CAD build for the part. Positions are in the model's coordinates, mm. A direction names the side the tool comes from. Coordinates: 2 decimals unless noted, no trailing zeros. Order: outer loops, then holes, each group sorted by start corner. A loop starts at its lowest first (then second) coordinate and runs counter-clockwise, first axis right, second up. Notation, with made-up numbers: (43, 74.25) - (86, 74.25) arc R21 cw to (86, 101.25) - close; hole circle Ø2 at (66, 27). An arc over 180 degrees is marked (long way). Use one line per item in the form item = value.
```python
from build123d import *

# Parameters (mm, degrees)
BOSS_EXTRUDE1_DEPTH = 10
SKETCH2_R           = 1.5
CUT_EXTRUDE1_DEPTH  = 107.852975625
BOSS_EXTRUDE2_DEPTH = 0.5
SKETCH5_R           = 3.25
CUT_EXTRUDE2_DEPTH  = 5
FILLET1_R           = 15


with BuildPart() as part:
    # Sketch1 → Boss-Extrude1 (new body)
    with BuildSketch(Plane(origin=(0, 0, 0), x_dir=(1, 0, 0), z_dir=(0, 1, 0))):
        with BuildLine():
            Line((0, 0), (10, 0))
            Line((10, 0), (58.28, 0))
            Line((58.28, 0), (58.28, 10))
            Line((58.28, 10), (10, 10))
            Line((10, 10), (10, 84))
            ThreePointArc((10, 84), (5, 89), (0, 84))
            Line((0, 84), (0, 10))
            Line((0, 10), (-5, 10))
            Line((-5, 10), (-5, 0))
            Line((-5, 0), (0, 0))
        make_face()
    extrude(amount=BOSS_EXTRUDE1_DEPTH)

    # Sketch2 → Cut-Extrude1 (cut, through all)
    with BuildSketch(Plane(origin=(0, 10, 0), x_dir=(1, 0, 0), z_dir=(0, 1, 0))):
        with Locations(Location((5, 84, 0), (0, 0, 270))):
            Circle(SKETCH2_R)
        with Locations(Location((5, 54, 0), (0, 0, 270))):
            Circle(SKETCH2_R)
    extrude(amount=-CUT_EXTRUDE1_DEPTH, mode=Mode.SUBTRACT)

    # Sketch4 → Boss-Extrude2 (add)
    with BuildSketch(Plane(origin=(0, 10, 0), x_dir=(1, 0, 0), z_dir=(0, 1, 0))):
        Polygon((3.358974359, 41.930004151), (4.794871795, 41.930004151), (4.794871795, 35.365901587), (7.051282051, 35.365901587), (7.051282051, 33.930004151), (3.358974359, 33.930004151), align=None)
    extrude(amount=BOSS_EXTRUDE2_DEPTH)

    # Sketch5 → Cut-Extrude2 (cut)
    with BuildSketch(Plane(origin=(0, 10, 0), x_dir=(1, 0, 0), z_dir=(0, 1, 0))):
        with Locations(Location((5, 84, 0), (0, 0, 270))):
            Circle(SKETCH5_R)
        with Locations(Location((5, 54, 0), (0, 0, 270))):
            Circle(SKETCH5_R)
    extrude(amount=-CUT_EXTRUDE2_DEPTH, mode=Mode.SUBTRACT)

    # Fillet1
    # the kernel refuses this fillet: 15 mm, written as the material it adds along each edge
    with BuildSketch(Plane(origin=(0, 0, -10), x_dir=(-1, 0, 0), z_dir=(0, 1, 0))) as fillet1_piece_1:
        with BuildLine():
            CenterArc((15, -11.180339887), FILLET1_R, 131.810314896, 48.189685104)
            Line((0, -11.180339887), (-0.3, -11.180339887))
            Line((-0.3, -11.180339887), (-0.3, 0))
            Line((-0.3, 0), (0, 0.3))
            ThreePointArc((0, 0.3), (2.5, 0.3), (4.8, 0.223606798))
            Line((4.8, 0.223606798), (5, 0))
        make_face()
    extrude(amount=10)
    with BuildSketch(Plane(origin=(10, 0, -10), x_dir=(1, 0, 0), z_dir=(0, 1, 0))) as fillet1_piece_2:
        with BuildLine():
            CenterArc((FILLET1_R, FILLET1_R), FILLET1_R, 180, 90)
            Line((0, FILLET1_R), (-FILLET1_R * 0.02, FILLET1_R))
            Line((-FILLET1_R * 0.02, FILLET1_R), (-FILLET1_R * 0.02, -FILLET1_R * 0.02))
            Line((-FILLET1_R * 0.02, -FILLET1_R * 0.02), (FILLET1_R, -FILLET1_R * 0.02))
            Line((FILLET1_R, -FILLET1_R * 0.02), (FILLET1_R, 0))
        make_face()
    extrude(amount=10)


solid = part.part
```
Item 1: Drop flat-ended pins along their axis: pin 1 (0.6 mm diameter, centred on y = 10.5, z = -38, fed in from +X); pin 2 (6 mm diameter, centred on y = 7.5, z = -63.5, fed in from -X); pin 3 (1 mm diameter, centred on y = 9, z = -45, fed in from +X). Give the stop position or say it passes through.
Derived:
pin_1 = 4.79
pin_2 = 0
pin_3 = 10
Item 2: Cut at A-A, the plane z = -54. Write the cut outline in (x, y).
Derived:
outline = (0, 0) - (3.5, 0) - (3.5, 5) - (1.75, 5) - (1.75, 10) - (0, 10) - close; (6.5, 0) - (10, 0) - (10, 10) - (8.25, 10) - (8.25, 5) - (6.5, 5) - close
Item 3: Two-plate mould, pull along Z, no slides. Class faces 5 (the face through (26, 5, 0)), 6 (the face through (42, 5, -10)), 7 (the face through (4.1, 2.5, -55.2)), 8 (the face through (10, 10, -22)): +Z half, -Z half, draft (parallel to the pull), parting line (faces both ways), or undercut.
Derived:
face_5 = +Z half
face_6 = -Z half
face_7 = undercut
face_8 = draft
Item 4: Cut at D-D, the plane y = 3. Write the cut outline in (x, z).
Derived:
outline = (-5, -10) arc R15 cw to (0, -21.18) - (0, -84) arc R5 ccw to (10, -84) - (10, -25) arc R15 cw to (25, -10) - (58.28, -10) - (58.28, 0) - (-5, 0) - close; hole circle Ø3 at (5, -84); hole circle Ø3 at (5, -54)
Item 5: Cut at C-C, the plane z = -41. Write the cut outline in (x, y).
Derived:
outline = (0, 0) - (10, 0) - (10, 10) - (4.79, 10) - (4.79, 10.5) - (3.36, 10.5) - (3.36, 10) - (0, 10) - close
Item 6: 3-axis set-ups, long thin cutter, end or side, ignore diameter. For faces 1 (the face through (6.5, 5, -83.3)), 2 (the face through (10, 5, -54)), 3 (the face through (0, 5, -53)), 4 (the face through (4, 10.5, -37)): which of +Z, -Z, +X, -X, +Y, -Y reach the whole face in a straight line?
Derived:
face_1 = +Y
face_2 = -Z, +X, +Y, -Y
face_3 = -Z, -X, +Y, -Y
face_4 = +Z, -Z, +X, -X, +Y
Item 7: Drill centre lines: line 1 (X direction, y = 7.5, z = -54); line 2 (Z direction, x = 3, y = 6); line 3 (Z direction, x = 33, y = 0.75). Where is each one in solid material? Low to high. Write a range as [from, to].
Derived:
line_1 = [0, 1.75], [8.25, 10]
line_2 = [-88.58, -86.56], [-81.44, -56.56], [-51.44, 0]
line_3 = [-10, 0]
Item 8: Cut at B-B, the plane y = 7.25. Write the cut outline in (x, z).
Derived:
outline = (-5, -10) arc R15 cw to (0, -21.18) - (0, -84) arc R5 ccw to (10, -84) - (10, -25) arc R15 cw to (25, -10) - (58.28, -10) - (58.28, 0) - (-5, 0) - close; hole circle Ø6.5 at (5, -84); hole circle Ø6.5 at (5, -54)
